Check sheet for the modelled part. Datum: model origin and axes. Units: mm. A direction names the side the tool comes from. Give positions to 0.01 mm unless a question says otherwise; leave off trailing zeros. Order: outer loops, then holes, each group sorted by start corner. A loop starts at its lowest first (then second) coordinate and runs counter-clockwise, first axis right, second up.
```python
from build123d import *

# Parameters (mm, degrees)
SKETCH_1_W          = 85.5
SKETCH_1_H          = 72.5
SKETCH_1_R          = 1.5
EXTRUDE_1_DEPTH     = 11.5
SKETCH_2_W          = 38.316664863
SKETCH_2_H          = 7.767596006
CUT_EXTRUDE_1_DEPTH = 3


with BuildPart() as part:
    # 草图1 → 凸台-拉伸1 (new body)
    with BuildSketch(Plane(origin=(0, 0, 0), x_dir=(1, 0, 0), z_dir=(0, 1, 0))):
        Rectangle(SKETCH_1_W, SKETCH_1_H)
        with Locations(Location((-40.2, 33.6, 0), (0, 0, 270))):
            Circle(SKETCH_1_R, mode=Mode.SUBTRACT)
        with Locations(Location((40.2, 33.6, 0), (0, 0, 90))):
            Circle(SKETCH_1_R, mode=Mode.SUBTRACT)
        with Locations(Location((40.2, -33.6, 0), (0, 0, 270))):
            Circle(SKETCH_1_R, mode=Mode.SUBTRACT)
        with Locations(Location((-40.2, -33.6, 0), (0, 0, 90))):
            Circle(SKETCH_1_R, mode=Mode.SUBTRACT)
    extrude(amount=EXTRUDE_1_DEPTH)

    # 草图2 → 切除-拉伸1 (cut)
    with BuildSketch(Plane.ZY.offset(42.75)):
        with Locations((5.239217441, 4.947785371)):
            Rectangle(SKETCH_2_W, SKETCH_2_H)
    extrude(amount=-CUT_EXTRUDE_1_DEPTH, mode=Mode.SUBTRACT)


solid = part.part
```
Q1. Material ranges on line 1 (X direction, y = 3.75, z = 33.6); line 2 (X direction, y = 9.5, z = 32.5); line 3 (X direction, y = 8, z = 22), recorded low to high.
Q2. Sectioned sample at A-A, the plane x = 40.2. Record the cut outline in (y, z), plus the area to 3 significant figures.
Q3. Draft check along Z on faces 1 (the flat face through (-1, 11.5, -1)), 2 (the flat face through (-1, 6, -36.25)), 3 (the flat face through (-41, 5, 24.398)). Enter one of: pulls with the +Z half, pulls with the -Z half, needs draft (parallel to the pull), parting line crosses it, or undercut.
Q4. Tool access check on faces 4 (the cylindrical face through (40.13, 5.67, -32.1)), 5 (the flat face through (-41, 5, -13.919)). Record the directions out of +Z, -Z, +X, -X, +Y, -Y that give a thin tool (end or side, any length) a straight path to the whole face; none if there is none.
Q5. Go/stop test with flat-tipped pins: P1, Ø1.5, axis at x = -29.5, z = 6.5, coming from the -Y side; P2, Ø2.5, axis at x = 40.2, z = -33.6, coming from the +Y side. Record where each tip stops, or that it passes through.
Q6. Sectioned sample at B-B, the plane z = 33.6. Record the cut outline in (x, y), plus the area to 3 significant figures.
Q7. Sectioned sample at C-C, the plane z = -10. Record the cut outline in (x, y), plus the area to 3 significant figures.
Filled in:
1. line 1: x = -42.75 to -41.7, -38.7 to 38.7, 41.7 to 42.75
1. line 2: x = -42.75 to -41.22, -39.18 to 39.18, 41.22 to 42.75
1. line 3: x = -39.75 to 42.75
2. outline: (0, -36.25) - (11.5, -36.25) - (11.5, -35.1) - (0, -35.1) - close; (0, -32.1) - (11.5, -32.1) - (11.5, 32.1) - (0, 32.1) - close; (0, 35.1) - (11.5, 35.1) - (11.5, 36.25) - (0, 36.25) - close
2. area: 765 mm2
3. face 1: needs draft
3. face 2: pulls with the -Z half
3. face 3: undercut
4. face 4: +Y, -Y
4. face 5: -X
5. P1: stops at y = 0
5. P2: passes through
6. outline: (-42.75, 0) - (-41.7, 0) - (-41.7, 11.5) - (-42.75, 11.5) - close; (-38.7, 0) - (38.7, 0) - (38.7, 11.5) - (-38.7, 11.5) - close; (41.7, 0) - (42.75, 0) - (42.75, 11.5) - (41.7, 11.5) - close
6. area: 914 mm2
7. outline: (-42.75, 0) - (42.75, 0) - (42.75, 11.5) - (-42.75, 11.5) - (-42.75, 8.83) - (-39.75, 8.83) - (-39.75, 1.06) - (-42.75, 1.06) - close
7. area: 960 mm2
